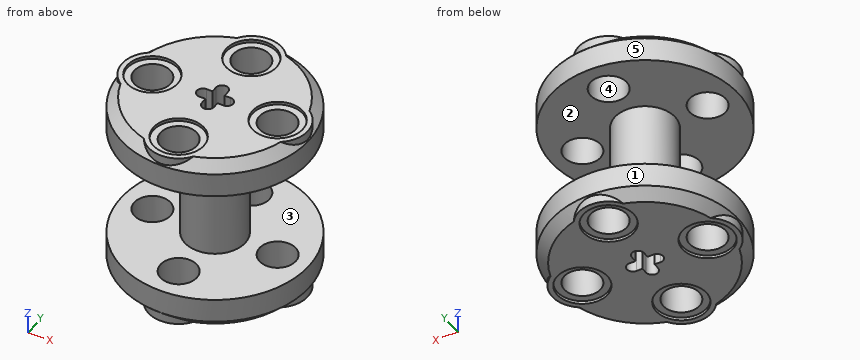
from build123d import *

# Parameters (mm, degrees)
SKETCH1_R           = 11.811
SKETCH1_R_2         = 2.286
EXTRUDE1_DEPTH      = 4.318
CHAMFER1_SIZE       = 1.27
SKETCH2_R           = 2.794
SKETCH2_R_2         = 2.306678084
SKETCH2_R_3         = 2.286
SKETCH2_R_4         = 2.290860138
EXTRUDE2_DEPTH      = 4.318
SKETCH3_R           = 3.81
EXTRUDE3_DEPTH      = 7.239
SKETCH4_W           = 1.524
SKETCH4_H           = 1.524
CUT_EXTRUDE1_DEPTH  = 12.557
SKETCH5_R           = 3.81
SKETCH5_R_2         = 2.286
BOSS_EXTRUDE3_DEPTH = 4.318
SKETCH6_R           = 3.81
SKETCH6_R_2         = 2.286
BOSS_EXTRUDE5_DEPTH = 4.318
SKETCH5_3_R         = 3.175
CUT_EXTRUDE2_DEPTH  = 0.381
SKETCH6_3_R         = 3.175
CUT_EXTRUDE3_DEPTH  = 0.381
CIRPATTERN1_COUNT   = 4


with BuildPart() as part:
    # Sketch1 → Extrude1 (new body)
    with BuildSketch(Plane.XY):
        Circle(SKETCH1_R)
        with Locations((0, 7.874)):
            Circle(SKETCH1_R_2, mode=Mode.SUBTRACT)
        with Locations((7.874, 0)):
            Circle(SKETCH1_R_2, mode=Mode.SUBTRACT)
        with Locations((0, -7.874)):
            Circle(SKETCH1_R_2, mode=Mode.SUBTRACT)
        with Locations((-7.874, 0)):
            Circle(SKETCH1_R_2, mode=Mode.SUBTRACT)
    extrude(amount=EXTRUDE1_DEPTH)

    # Chamfer1
    chamfer1_edges = [part.edges().sort_by_distance(p)[0] for p in [
        (-11.811, 0, 4.318),
    ]]
    chamfer(chamfer1_edges, length=CHAMFER1_SIZE)

    # Sketch2 → Extrude2 (add)
    with BuildSketch(Plane.XY.offset(4.318)):
        with Locations((0, 7.874)):
            Circle(SKETCH2_R)
        with Locations((0, 7.874)):
            Circle(SKETCH2_R_2, mode=Mode.SUBTRACT)
        with Locations((-7.874, 0)):
            Circle(SKETCH2_R)
        with Locations((-7.874, 0)):
            Circle(SKETCH2_R_3, mode=Mode.SUBTRACT)
        with Locations((0, -7.874)):
            Circle(SKETCH2_R)
        with Locations((0, -7.874)):
            Circle(SKETCH2_R_4, mode=Mode.SUBTRACT)
        with Locations((7.874, 0)):
            Circle(SKETCH2_R)
        with Locations((7.874, 0)):
            Circle(SKETCH2_R_3, mode=Mode.SUBTRACT)
    extrude(amount=-EXTRUDE2_DEPTH)

    # Sketch3 → Extrude3 (add)
    with BuildSketch(Plane(origin=(0, 0, 0), x_dir=(-1, 0, 0), z_dir=(0, 0, -1))):
        Circle(SKETCH3_R)
    extrude(amount=EXTRUDE3_DEPTH)

    # Sketch4 → Cut-Extrude1 (cut, through all)
    with BuildSketch(Plane.XY.offset(4.318)):
        with BuildLine():
            Line((-0.762, 0.762), (-1.524, 0.762))
            ThreePointArc((-1.524, 0.762), (-2.286, 0), (-1.524, -0.762))
            Line((-1.524, -0.762), (-0.762, -0.762))
            Line((-0.762, -0.762), (-0.762, 0.762))
        make_face()
        with BuildLine():
            Line((-0.762, 1.524), (-0.762, 0.762))
            Line((-0.762, 0.762), (0.762, 0.762))
            Line((0.762, 0.762), (0.762, 1.524))
            ThreePointArc((0.762, 1.524), (0, 2.286), (-0.762, 1.524))
        make_face()
        with BuildLine():
            Line((1.524, 0.762), (0.762, 0.762))
            Line((0.762, 0.762), (0.762, -0.762))
            Line((0.762, -0.762), (1.524, -0.762))
            ThreePointArc((1.524, -0.762), (2.286, 0), (1.524, 0.762))
        make_face()
        Rectangle(SKETCH4_W, SKETCH4_H)
        with BuildLine():
            Line((0.762, -0.762), (-0.762, -0.762))
            Line((-0.762, -0.762), (-0.762, -1.524))
            ThreePointArc((-0.762, -1.524), (0, -2.286), (0.762, -1.524))
            Line((0.762, -1.524), (0.762, -0.762))
        make_face()
    extrude(amount=-CUT_EXTRUDE1_DEPTH, mode=Mode.SUBTRACT)

    # Mirror1: part across plane


with BuildPart() as part_1:
    add(part.part)
    add(part.part.mirror(Plane.XY.offset(-7.239)))

    # Sketch5 → Boss-Extrude3 (add)
    with BuildSketch(Plane.XY.offset(4.318)):
        with Locations((0, 7.874)):
            Circle(SKETCH5_R)
        with Locations((0, 7.874)):
            Circle(SKETCH5_R_2, mode=Mode.SUBTRACT)
    boss_extrude3 = extrude(amount=-BOSS_EXTRUDE3_DEPTH)

    # Sketch6 → Boss-Extrude5 (add)
    with BuildSketch(Plane(origin=(0, 0, -18.796), x_dir=(-1, 0, 0), z_dir=(0, 0, -1))):
        with Locations((0, 7.874)):
            Circle(SKETCH6_R)
        with Locations((0, 7.874)):
            Circle(SKETCH6_R_2, mode=Mode.SUBTRACT)
    boss_extrude5 = extrude(amount=-BOSS_EXTRUDE5_DEPTH)

    # Sketch5_3 → Cut-Extrude2 (cut)
    with BuildSketch(Plane.XY.offset(4.318)):
        with Locations((0, 7.874)):
            Circle(SKETCH5_3_R)
    cut_extrude2 = extrude(amount=-CUT_EXTRUDE2_DEPTH, mode=Mode.SUBTRACT)

    # Sketch6_3 → Cut-Extrude3 (cut)
    with BuildSketch(Plane(origin=(0, 0, -18.796), x_dir=(-1, 0, 0), z_dir=(0, 0, -1))):
        with Locations((0, 7.874)):
            Circle(SKETCH6_3_R)
    cut_extrude3 = extrude(amount=-CUT_EXTRUDE3_DEPTH, mode=Mode.SUBTRACT)

    # CirPattern1: Boss-Extrude3, Boss-Extrude5, Cut-Extrude2, Cut-Extrude3 ×4 about axis
    cirpattern1_axis = Axis((0, 0, 0), (0, 0, 1))
    for i in range(1, CIRPATTERN1_COUNT):
        add(boss_extrude3.rotate(cirpattern1_axis, i * 360 / CIRPATTERN1_COUNT))
        add(boss_extrude5.rotate(cirpattern1_axis, i * 360 / CIRPATTERN1_COUNT))
        add(cut_extrude2.rotate(cirpattern1_axis, i * 360 / CIRPATTERN1_COUNT), mode=Mode.SUBTRACT)
        add(cut_extrude3.rotate(cirpattern1_axis, i * 360 / CIRPATTERN1_COUNT), mode=Mode.SUBTRACT)


solid = part_1.part
Can you work these out from the model? Positions are in its coordinate system, mm. Face numbers are marked on the shaded views. A direction names the side the tool comes from. Coordinates: 2 decimals unless noted, no trailing zeros. Write each loop counter-clockwise with the first axis right and the second up, starting at its lowest first coordinate (ties: lowest second). Pieces come first, ordered by that corner, then holes. Notation, with made-up numbers: (70.5, 87.5) -> (111.5, 87.5) arc R23 cw to (111.5, 125.5) -> close; hole circle Ø3 at (-19.75, 23.25). An arc over 180 degrees is marked (long way). Write each question's results on one line, items separated by ' | '. Start each with the question number.
Item 1: If we section it at B-B, the plane z = 2.25: Write out the boundary of the cut face in (x, y), and give its area (3 significant figures).
Item 2: If we section it at A-A, the plane z = -9.25: Write out the boundary of the cut face in (x, y), and give its area (3 significant figures).
Item 3: Thinking about a two-plate mould opening in Y: for the marked faces 3, 4 and 5, which applies, released by +Y, released by -Y, zero draft, split by the parting line, or undercut?
Item 4: I'm going to push flat-ended pins straight in: P1, Ø5.5, axis at x = 0, y = -7.874, coming from the -Z side (3 decimals); P2, Ø4, axis at x = 0, y = 7.874, coming from the -Z side; P3, Ø2, axis at y = -3, z = -15, coming from the -X side; P4, Ø12, axis at x = 9.5, z = -3, coming from the -Y side. Where does each tip first touch, or does it pass through?
Item 5: Please list where these lines run through material, in increasing order: probe 1 along X at (y, z) = (0, -18.7); probe 2 along Z at (x, y) = (-7.5, 5.75); probe 3 along Z at (x, y) = (3.5, 10.75).
Item 6: On a 3-axis mill with a long thin cutter (end or side, diameter ignored), from which of +Z, -Z, +X, -X, +Y, -Y can I reach the whole of each face in a straight line? I mean the marked faces 1 and 2. Say none if no direction works.
Item 7: If we section it at C-C, the plane y = 0: Count the separate pieces of the cut face and the enclosed holes in it, and give its area (3 significant figures).
Answer block:
1) outline: circle Ø23.62 at (0, 0); hole circle Ø4.57 at (-7.87, 0); hole circle Ø4.57 at (0, -7.87); hole circle Ø4.57 at (0, 7.87); hole (-1.52, -0.76) -> (-0.76, -0.76) -> (-0.76, -1.52) arc R0.76 ccw to (0.76, -1.52) -> (0.76, -0.76) -> (1.52, -0.76) arc R0.76 ccw to (1.52, 0.76) -> (0.76, 0.76) -> (0.76, 1.52) arc R0.76 ccw to (-0.76, 1.52) -> (-0.76, 0.76) -> (-1.52, 0.76) arc R0.76 ccw to start; hole circle Ø4.57 at (7.87, 0) | area: 362 mm²
2) outline: circle Ø7.62 at (0, 0); hole (-1.52, -0.76) -> (-0.76, -0.76) -> (-0.76, -1.52) arc R0.76 ccw to (0.76, -1.52) -> (0.76, -0.76) -> (1.52, -0.76) arc R0.76 ccw to (1.52, 0.76) -> (0.76, 0.76) -> (0.76, 1.52) arc R0.76 ccw to (-0.76, 1.52) -> (-0.76, 0.76) -> (-1.52, 0.76) arc R0.76 ccw to start | area: 35.0 mm²
3) face 3: zero draft | face 4: undercut | face 5: split by the parting line
4) P1: z = -18.415 | P2: through | P3: x = -11.64 | P4: y = -11
5) probe 1: -11.68 to -11.05, -4.7 to -2.29, 2.29 to 4.7, 11.05 to 11.68 | probe 2: -18.8 to -14.48, 0 to 4.32 | probe 3: -18.03 to -14.48, 0 to 3.55
6) face 1: +Z, -Z | face 2: none
7) separate pieces: 6 | enclosed holes: 0 | area: 126 mm²
